Can you work these out from the model? Positions are in its coordinate system, mm. Give positions to 0.01 mm unless a question says otherwise; leave off trailing zeros. Order: outer loops, then holes, each group sorted by start corner. A loop starts at its lowest first (then second) coordinate and runs counter-clockwise, first axis right, second up. Notation, with made-up numbers: (73, 58.5) - (131, 58.5) arc R17 cw to (131, 80.5) - close; hole circle Ø6 at (22.5, 21). An arc over 180 degrees is marked (long way). Use one line per item in the form item = value. Start each with the question number.
1) For pin 1 (12.5 mm diameter, centred on x = 123.5, y = 221, fed in from +Z) (3 decimals); pin 2 (6.5 mm diameter, centred on y = 123.5, z = 9, fed in from -X); pin 3 (10 mm diameter, centred on x = 66, y = 49.5, fed in from +Z) (3 decimals), each with a flat end and sliding along its axis, tell me the tip position at first contact or that it passes through.
2) Suppose I cut it at C-C, the plane z = 24. Write out the boundary of the cut face in (x, y), and give its area (3 significant figures).
3) Suppose I cut it at A-A, the plane z = 7. Write out the boundary of the cut face in (x, y), and give its area (3 significant figures).
4) Please list where these lines run through material, in increasing order: probe 1 along Z at (x, y) = (83.5, 101) (3 decimals); probe 2 along X at (y, z) = (152, 6.5); probe 3 along Y at (x, z) = (14.5, 15.75).
5) Suppose I cut it at B-B, the plane x = 19.05. Write out the boundary of the cut face in (y, z) (3 decimals).
6) Suppose I cut it at D-D, the plane y = 229.5. Write out the boundary of the cut face in (x, z) (3 decimals).
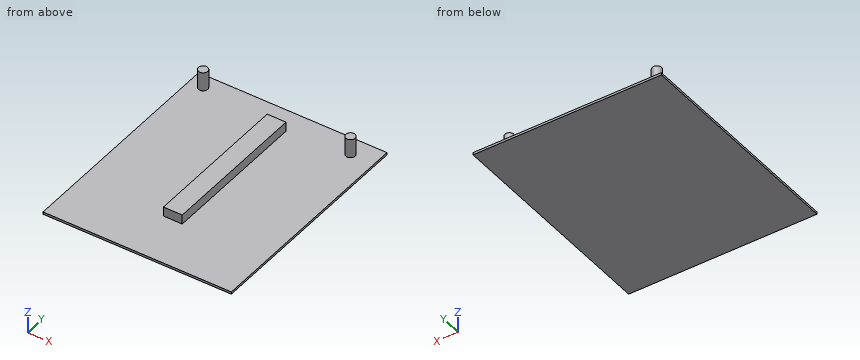
```python
from build123d import *

# Parameters (mm, degrees)
F0_W     = 254
F0_H     = 304.8
F1_DEPTH = 3.175
F2_W     = 25.4
F2_H     = 203.2
F3_DEPTH = 12.7
F4_R     = 6.35
F5_DEPTH = 25.4


with BuildPart() as f1:
    # F0 (on Top) → F1 (new body)
    with BuildSketch(Plane.XY):
        with Locations((127, 152.4)):
            Rectangle(F0_W, F0_H)
    extrude(amount=F1_DEPTH)

    # F2 (on face) → F3 (join)
    with BuildSketch(Plane.XY.offset(3.175)):
        with Locations((127, 171.425429)):
            Rectangle(F2_W, F2_H)
    extrude(amount=F3_DEPTH)

    # F4 (on face) → F5 (join)
    with BuildSketch(Plane.XY.offset(3.175)):
        with Locations((222.25, 279.4)):
            Circle(F4_R)
        with Locations((19.05, 285.75)):
            Circle(F4_R)
    extrude(amount=F5_DEPTH)


solid = f1.part
```
Result sheet:
q1.pin_1 = 15.875
q1.pin_2 = 114.3
q1.pin_3 = 3.175
q2.outline = circle Ø12.7 at (19.05, 285.75); circle Ø12.7 at (222.25, 279.4)
q2.area = 253 mm²
q3.outline = circle Ø12.7 at (19.05, 285.75); (114.3, 69.83) - (139.7, 69.83) - (139.7, 273.03) - (114.3, 273.03) - close; circle Ø12.7 at (222.25, 279.4)
q3.area = 5,410 mm²
q4.probe_1 = 0 to 3.175
q4.probe_2 = 114.3 to 139.7
q4.probe_3 = 281.32 to 290.18
q5.outline = (0, 0) - (304.8, 0) - (304.8, 3.175) - (292.1, 3.175) - (292.1, 28.575) - (279.4, 28.575) - (279.4, 3.175) - (0, 3.175) - close
q6.outline = (0, 0) - (254, 0) - (254, 3.175) - (139.7, 3.175) - (139.7, 15.875) - (114.3, 15.875) - (114.3, 3.175) - (0, 3.175) - close
